Autodesk Inventor part; units mm, degrees
ref_plane "YZ Plane" through (0, 0, 0) normal (1, 0, 0) x (0, 1, 0)
ref_plane "XZ Plane" through (0, 0, 0) normal (0, 1, 0) x (-1, 0, 0)
ref_plane "XY Plane" through (0, 0, 0) normal (0, 0, 1) x (1, 0, 0)
sketch "Эскиз1" plane through (0, 0, 0) normal (0, 0, 1) x (1, 0, 0)
  line L0 (31.5, -28.5) -> (-31.5, -28.5)
  line L1 (-31.5, -28.5) -> (-31.5, 28.5)
  line L2 (-31.5, 28.5) -> (31.5, 28.5)
  line L3 (31.5, 28.5) -> (31.5, -28.5)
  line L4 (31.5, -28.5) -> (-31.5, 28.5) construction
  line L5 (-31.5, -28.5) -> (31.5, 28.5) construction
  line L6 (-31.5, 28.5) -> (31.5, 28.5)
  line L7 (31.5, 28.5) -> (31.5, 25.5)
  line L8 (31.5, 25.5) -> (-31.5, 25.5)
  line L9 (-31.5, 25.5) -> (-31.5, 28.5)
  line L10 (-31.5, 28.5) -> (-28.5, 28.5)
  line L11 (-28.5, 28.5) -> (-28.5, -28.5)
  line L12 (-28.5, -28.5) -> (-31.5, -28.5)
  line L13 (-31.5, -28.5) -> (-31.5, 28.5)
  line L14 (31.5, 28.5) -> (28.5, 28.5)
  line L15 (28.5, 28.5) -> (28.5, -28.5)
  line L16 (28.5, -28.5) -> (31.5, -28.5)
  line L17 (31.5, -28.5) -> (31.5, 28.5)
  line L18 (11.5, -8.5) -> (-11.5, -8.5)
  line L19 (-11.5, -8.5) -> (-11.5, 14.5)
  line L20 (-11.5, 14.5) -> (11.5, 14.5)
  line L21 (11.5, 14.5) -> (11.5, -8.5)
  line L22 (11.5, -8.5) -> (-11.5, 14.5) construction
  line L23 (-11.5, -8.5) -> (11.5, 14.5) construction
  line L24 (-11.5, 14.5) -> (10, 14.5)
  line L25 (10, 14.5) -> (10, -28.5)
  line L26 (10, -28.5) -> (-11.5, -28.5)
  line L27 (-11.5, -28.5) -> (-11.5, 14.5)
  line L28 (-31.5, 28.5) -> (-28.5, 28.5)
  line L29 (-28.5, 28.5) -> (-28.5, 8.5)
  line L30 (-28.5, 8.5) -> (-31.5, 8.5)
  line L31 (-31.5, 8.5) -> (-31.5, 28.5)
  line L32 (-31.5, 8.5) -> (-28.5, 8.5)
  line L33 (-28.5, 8.5) -> (-28.5, -3.5)
  line L34 (-28.5, -3.5) -> (-31.5, -3.5)
  line L35 (-31.5, -3.5) -> (-31.5, 8.5)
  line L36 (0, 0) -> (0, 3)
  line L37 (28.5, 8.5) -> (31.5, 8.5)
  line L38 (28.5, -3.5) -> (31.5, -3.5)
  line L39 (-20, -22.5) -> (20, -22.5)
  line L40 (20, -22.5) -> (20, 28.5)
  line L41 (20, 28.5) -> (-20, 28.5)
  line L42 (-20, 28.5) -> (-20, -22.5)
  line L43 (-20, -22.5) -> (20, 28.5) construction
  line L44 (20, -22.5) -> (-20, 28.5) construction
  line L45 (-28.5, 2.5) -> (28.5, 2.5)
  line L46 (35, -28.5) -> (-35, -28.5)
  line L47 (-35, -28.5) -> (-35, 28.5)
  line L48 (-35, 28.5) -> (35, 28.5)
  line L49 (35, 28.5) -> (35, -28.5)
  line L50 (35, -28.5) -> (-35, 28.5) construction
  line L51 (-35, -28.5) -> (35, 28.5) construction
  line L52 (-28.5, 2.5) -> (-30, 2.5)
  circle A0 centre (-30, 2.5) radius 1.5
  circle A1 centre (30, 2.5) radius 1.5
  line L53 (-31.5, 8.5) -> (-35, 8.5)
  line L54 (-35, 8.5) -> (-35, -3.5)
  line L55 (-35, -3.5) -> (-31.5, -3.5)
  line L56 (-31.5, -3.5) -> (-31.5, 8.5)
  line L57 (31.5, -3.5) -> (35, -3.5)
  line L58 (35, -3.5) -> (35, 8.5)
  line L59 (35, 8.5) -> (31.5, 8.5)
  line L60 (31.5, 8.5) -> (31.5, -3.5)
  point P0 (-31.5, -3.5)
  point P1 (-11.5, -28.5)
  point P2 (-28.5, 25.5)
  point P3 (-31.5, 8.5)
  point P4 (-20, 25.5)
  point P5 (28.5, -3.5)
  point P6 (31.5, -3.5)
  point P7 (28.5, 8.5)
  point P8 (28.5, 25.5)
  point P9 (20, 25.5)
  point P10 (20, 28.5)
  point P11 (10, -8.5)
  dimension "d0" = 63
  dimension "d1" = 57
  dimension "d2" = 3
  dimension "d3" = 3
  dimension "d4" = 3
  dimension "d5" = 23
  dimension "d6" = 23
  dimension "d7" = 20
  dimension "d8" = 12
  dimension "d12" = 40
  dimension "d13" = 70
extrude "Выдавливание1" add sketch "Эскиз1" along normal blind 3 contours L0 L25 L39 L40 L45 L15 | L38 L15 A1 L3 | L3 L59 L49 L57 | A1 L15 L37 L3 | L0 L11 L45 L42 L39 L27 | L25 L18 L21 L45 L40 L39 | L45 L40 L8 L15 | L39 L42 L45 L19 L27 | L25 L45 L21 L18 | L45 L21 L20 L19 L42 L8 L40 | L34 L1 A0 L11 | L25 L20 L21 L45 | L8 L42 L2 L40 | L55 L47 L53 L1 | A0 L1 L30 L11 | L11 L8 L42 L45
properties part number "бок"
Source: CAD feature listing. Evaluate the final solid. Frame: model axes, mm. A direction names the side the tool comes from. Round coordinates to 2 decimals unless told otherwise and drop trailing zeros. Order: outer loops, then holes, each group sorted by start corner. A loop starts at its lowest first (then second) coordinate and runs counter-clockwise, first axis right, second up. Notation, with made-up numbers: (23.5, 38) -> (49.5, 38) arc R20 ccw to (49.5, 56) -> close; hole circle Ø10 at (52, 65.25). An arc over 180 degrees is marked (long way). Answer as CSV lines item,"result".
Item 1: Pull-direction query (X, two-part tool) for faces 5 (the face through (-28.5, -16, 1)), 6 (the face through (35, 3, 1)), 7 (the face through (32, -3.5, 1)), 8 (the face through (10, -7, 1)); classes: pulls with the +X half, pulls with the -X half, needs draft (parallel to the pull), parting line crosses it, or undercut.
A:
face 5,"pulls with the -X half"
face 6,"pulls with the +X half"
face 7,"needs draft"
face 8,"undercut"
Item 2: Line query: L1, parallel to X at y = 2.5, z = 1.85; L2, parallel to Y at x = -30, z = 1.8; L3, parallel to X at y = -19.5, z = 2.75. Output: solid intervals per line, ascending.
A:
L1,"-35 to -31.5, -28.5 to -11.5, 10 to 28.5, 31.5 to 35"
L2,"-3.5 to 1, 4 to 8.5"
L3,"-28.5 to -11.5, 10 to 28.5"
Item 3: Reachability of faces 1 (the face through (-32, 8.5, 1)), 2 (the face through (-1, 14.5, 1)), 3 (the face through (32, 8.5, 1)), 4 (the face through (28.5, -16, 1)) from +Z, -Z, +X, -X, +Y, -Y: full face, straight path, thin tool, end or side. Return the list, or none.
A:
face 1,"+Z, -Z, -X, +Y"
face 2,"+Z, -Z, -Y"
face 3,"+Z, -Z, +X, +Y"
face 4,"+Z, -Z, +X, -Y"
Item 4: Pin query (flat end, axial travel): pin 1 Ø1.5 at (x, z) = (32.5, 1) entering from +Y; pin 2 Ø1.5 at (x, z) = (26, 1.5) entering from +Y; pin 3 Ø0.9 at (y, z) = (27.5, 1) entering from +X. Return the tip coordinate at first contact, or that it passes through.
A:
pin 1,"y = 8.5"
pin 2,"y = 25.5"
pin 3,"x = 20"
Item 5: Section C-C, the plane z = 2.25. Return loops of the section in (x, y).
A:
outline,"(-35, -3.5) -> (-28.5, -3.5) -> (-28.5, -28.5) -> (-11.5, -28.5) -> (-11.5, 14.5) -> (10, 14.5) -> (10, -28.5) -> (28.5, -28.5) -> (28.5, -3.5) -> (35, -3.5) -> (35, 8.5) -> (28.5, 8.5) -> (28.5, 25.5) -> (20, 25.5) -> (20, 28.5) -> (-20, 28.5) -> (-20, 25.5) -> (-28.5, 25.5) -> (-28.5, 8.5) -> (-35, 8.5) -> close; hole circle Ø3 at (-30, 2.5); hole circle Ø3 at (30, 2.5)"
Item 6: Section D-D, the plane x = -2.5. Return loops of the section in (y, z), plus the area to 3 significant figures.
A:
outline,"(14.5, 0) -> (28.5, 0) -> (28.5, 3) -> (14.5, 3) -> close"
area,"42.0 mm²"
Item 7: Section B-B, the plane y = 2.5. Return loops of the section in (x, z).
A:
outline,"(-35, 0) -> (-31.5, 0) -> (-31.5, 3) -> (-35, 3) -> close; (-28.5, 0) -> (-11.5, 0) -> (-11.5, 3) -> (-28.5, 3) -> close; (10, 0) -> (28.5, 0) -> (28.5, 3) -> (10, 3) -> close; (31.5, 0) -> (35, 0) -> (35, 3) -> (31.5, 3) -> close"
Item 8: Section A-A, the plane y = -16. Return loops of the section in (x, z), plus the area to 4 significant figures.
A:
outline,"(-28.5, 0) -> (-11.5, 0) -> (-11.5, 3) -> (-28.5, 3) -> close; (10, 0) -> (28.5, 0) -> (28.5, 3) -> (10, 3) -> close"
area,"106.5 mm²"
